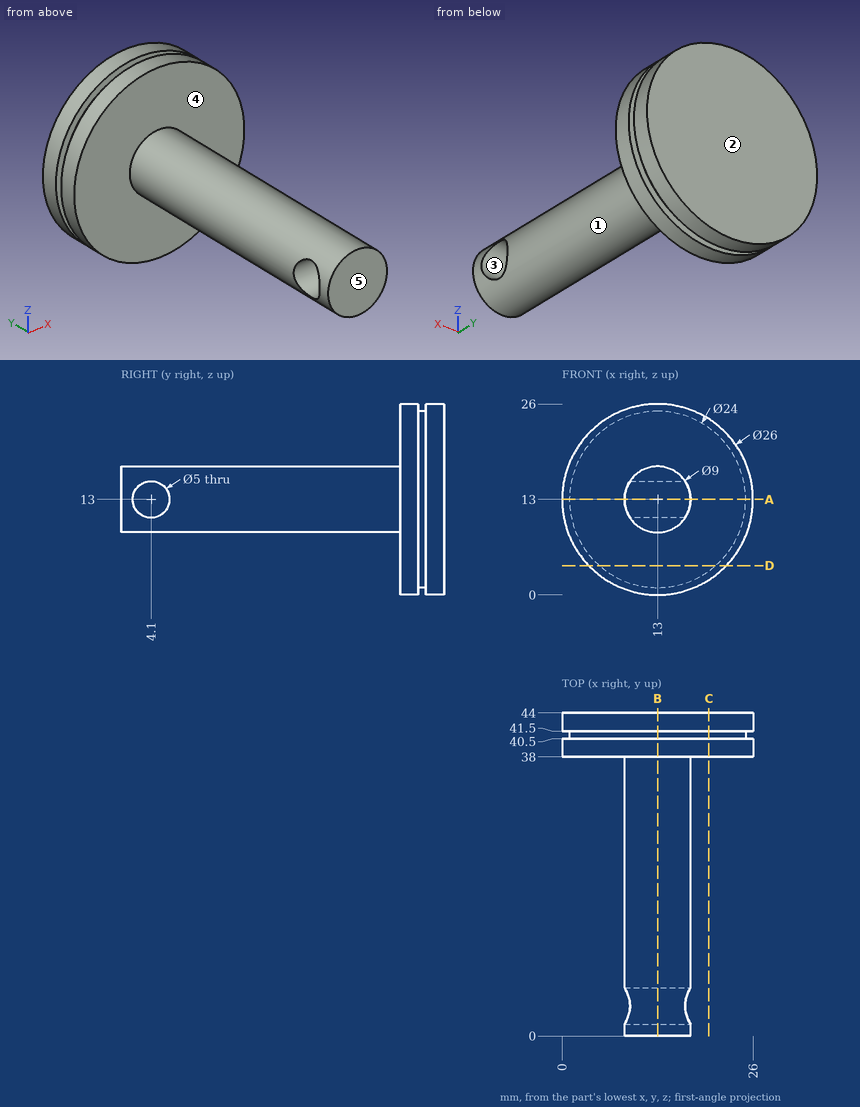
Study the drawing (mm; zero at the part's minimum x, y, z) and answer. A direction names the side the tool comes from. Round coordinates to 2 decimals unless told otherwise and drop trailing zeros. Order: outer loops, then holes, each group sorted by start corner. A loop starts at its lowest first (then second) coordinate and runs counter-clockwise, first axis right, second up. Notation, with made-up numbers: (25.25, 62) - (33.25, 62) arc R26 ccw to (33.25, 89) - close; hole circle Ø7 at (64.5, -38). An arc over 180 degrees is marked (long way). Use one line per item in the form item = value. Start each with the question number.
(1) The part is cut by section A-A (z = 13). Give the vertices of the cut face in (x, y), then the cut area to 3 significant figures.
(2) For the marked faces 4 and 5, determine the directions among +Z, -Z, +X, -X, +Y, -Y from which every point of the face is accessible in a straight line to the end or side of a thin tool.
(3) Find the intervals of material crossed by line 1 along Y through (x, z) = (13.75, 13); line 2 along Y through (x, z) = (2, 14.25); line 3 along X through (y, z) = (12.5, 16.25), in increasing order. Write a range as from..to.
(4) The part is cut by section D-D (z = 4). Give the vertices of the cut face in (x, y).
(5) The part is cut by section C-C (x = 20). Give the vertices of the cut face in (y, z).
(6) Determine the mould class of the marked faces 1, 2 and 3 for opening direction Z: +Z half, -Z half, draft (parallel to the pull), parting line (faces both ways), or undercut.
(7) The part is cut by section B-B (x = 13). Give the vertices of the cut face in (y, z), then the cut area to 3 significant figures.
(8) Flat-ended cylindrical pins translate along their axes: pin 1 Ø10 at (y, z) = (29, 6.5) entering from +X; pin 2 Ø6 at (y, z) = (31.5, 7.5) entering from -X; pin 3 Ø1.5 at (y, z) = (16, 15) entering from +X. Find the tip coordinate at first contact, or state that the pin passes through.
Checked values:
q1.outline = (0, 38) - (8.5, 38) - (8.5, 6.6) - (17.5, 6.6) - (17.5, 38) - (26, 38) - (26, 40.5) - (25, 40.5) - (25, 41.5) - (26, 41.5) - (26, 44) - (0, 44) - (0, 41.5) - (1, 41.5) - (1, 40.5) - (0, 40.5) - close; (8.5, 0) - (17.5, 0) - (17.5, 1.6) - (8.5, 1.6) - close
q1.area = 451 mm^2
q2.face_4 = -Y
q2.face_5 = +Z, -Z, +X, -X, -Y
q3.line_1 = 0..1.6, 6.6..44
q3.line_2 = 38..44
q3.line_3 = 9.89..16.11
q4.outline = (3.62, 38) - (22.38, 38) - (22.38, 40.5) - (20.94, 40.5) - (20.94, 41.5) - (22.38, 41.5) - (22.38, 44) - (3.62, 44) - (3.62, 41.5) - (5.06, 41.5) - (5.06, 40.5) - (3.62, 40.5) - close
q5.outline = (38, 2.05) - (40.5, 2.05) - (40.5, 3.25) - (41.5, 3.25) - (41.5, 2.05) - (44, 2.05) - (44, 23.95) - (41.5, 23.95) - (41.5, 22.75) - (40.5, 22.75) - (40.5, 23.95) - (38, 23.95) - close
q6.face_1 = parting line
q6.face_2 = draft
q6.face_3 = undercut
q7.outline = (0, 8.5) - (38, 8.5) - (38, 0) - (40.5, 0) - (40.5, 1) - (41.5, 1) - (41.5, 0) - (44, 0) - (44, 26) - (41.5, 26) - (41.5, 25) - (40.5, 25) - (40.5, 26) - (38, 26) - (38, 17.5) - (0, 17.5) - close; hole circle Ø5 at (4.1, 13)
q7.area = 476 mm^2
q8.pin_1 = 17.24
q8.pin_2 = 9.26
q8.pin_3 = 17.32
